Can you work these out from the model? Positions are in its coordinate system, mm. A direction names the side the tool comes from. Coordinates: 2 decimals unless noted, no trailing zeros. Write each loop counter-clockwise with the first axis right and the second up, starting at its lowest first coordinate (ties: lowest second). Pieces come first, ordered by that corner, then holes. Notation, with made-up numbers: M 68.25,-7.75 L 106.25,-7.75 A19 cw 106.25,3.25 Z; hole C 0,57.5 d2. An arc over 180 degrees is marked long. Use one line per item in the form item = value. Start each with the question number.
```python
from build123d import *

# Parameters (mm, degrees)
F0_W     = 180
F0_H     = 80
F1_DEPTH = 85
F3_DEPTH = 85.001
F5_DEPTH = 85.001


with BuildPart() as f1:
    # F0 (on Front) → F1 (new body)
    with BuildSketch(Plane.XZ):
        with Locations((4.7223418951, 11.9884983084)):
            Rectangle(F0_W, F0_H)
    extrude(amount=F1_DEPTH)

    # F2 (on face) → F3 (cut, through all)
    with BuildSketch(Plane.XZ.offset(85)):
        Polygon((-46.0070036352, -28.0115016916), (-85.2776581049, 51.9884983084), (-85.2776581049, -28.0115016916), align=None)
        Polygon((94.7223418951, -28.0115016916), (94.7223418951, 51.9884983084), (55.2294403315, -28.0115016916), align=None)
    extrude(amount=-F3_DEPTH, mode=Mode.SUBTRACT)

    # F4 (on face) → F5 (cut, through all)
    with BuildSketch(Plane.XZ.offset(85)):
        Polygon((-74.7092828557, 46.072713804), (-67.7043439121, 31.8026405634), (76.6995772719, 31.8026405634), (83.6467270564, 46.072713804), align=None)
        Polygon((73.4329734772, 25.2924152588), (-64.5085838063, 25.2924152588), (-38.3425875008, -28.0115016916), (46.6869287193, -28.0115016916), align=None)
    extrude(amount=-F5_DEPTH, mode=Mode.SUBTRACT)


solid = f1.part
```
1) Suppose I cut it at A-A on x = -33. Please give me the cut outline in (y, z).
2) Suppose I cut it at C-C on z = 5.5. Please give me the cut outline in (x, y).
3) Suppose I cut it at D-D on x = 51.5. Please give me the cut outline in (y, z), and give its area (3 significant figures).
4) Please list where these lines run through material, in increasing order: line 1 (Z direction, x = 64, y = -24); line 2 (Z direction, x = 16, y = -77); line 3 (Z direction, x = -43, y = -57).
5) Will these pins go through, and if not, where does the flat tip stop? pin 1 Ø12 at (y, z) = (-66, 18) entering from +X; pin 2 Ø10 at (y, z) = (-27.5, -0.5) entering from -X; pin 3 Ø6 at (y, z) = (-10, 42.5) entering from +X; pin 4 Ø5 at (x, y) = (45.5, -35.5) entering from -Z.
6) Suppose I cut it at B-B on y = -58. Please give me the cut outline in (x, z), and give its area (3 significant figures).
7) Which directions (+Z, -Z, +X, -X, +Y, -Y) give clear straight access to the entire face, cutting with the end or side of a thin tool? Please do faces 1 (the face through (-65.37, -43.1, 11.43)), 2 (the face through (3, -43, 31.803)).
8) If we mould it in two halves opening along Z, with no side actions, what happens to faces 3 (the face through (80.125, -43.095, 38.838)), 4 (the face through (3, -42, 51.988)), 5 (the face through (75.252, -43.095, 12.548))? For each: +Z half, -Z half, draft (parallel to the pull), parting line (faces both ways), or undercut.
Computed values:
q1.outline = M -85,25.29 L 0,25.29 L 0,31.8 L -85,31.8 Z; M -85,46.07 L 0,46.07 L 0,51.99 L -85,51.99 Z
q2.outline = M -62.46,-85 L -54.79,-85 L -54.79,0 L -62.46,0 Z; M 63.5,-85 L 71.77,-85 L 71.77,0 L 63.5,0 Z
q3.outline = M -85,-28.01 L 0,-28.01 L 0,-18.42 L -85,-18.42 Z; M -85,25.29 L 0,25.29 L 0,31.8 L -85,31.8 Z; M -85,46.07 L 0,46.07 L 0,51.99 L -85,51.99 Z
q3.area = 1,870 mm²
q4.line_1 = -10.25 to 6.49, 25.29 to 31.8, 46.07 to 51.99
q4.line_2 = 25.29 to 31.8, 46.07 to 51.99
q4.line_3 = -28.01 to -18.52, 25.29 to 31.8, 46.07 to 51.99
q5.pin_1 = 80.91
q5.pin_2 = -61.97
q5.pin_3 = 91.52
q5.pin_4 = -28.01
q6.outline = M -85.28,51.99 L -46.01,-28.01 L -38.34,-28.01 L -64.51,25.29 L 73.43,25.29 L 46.69,-28.01 L 55.23,-28.01 L 94.72,51.99 Z; hole M -74.71,46.07 L -67.7,31.8 L 76.7,31.8 L 83.65,46.07 Z
q6.area = 3,150 mm²
q7.face_1 = -Z, -X, +Y, -Y
q7.face_2 = +Y, -Y
q8.face_3 = undercut
q8.face_4 = +Z half
q8.face_5 = -Z half
